Here's how the part is built. I have some questions about the finished solid (model axes, mm). Face numbers are marked on the shaded views. A direction names the side the tool comes from. Give positions to 0.01 mm unless a question says otherwise; leave off trailing zeros. Loops run counter-clockwise (first coordinate to the right, second up) from the corner with the lowest first, then second, coordinate; pieces in that order, holes last. Notation, with made-up numbers: M 52,85 L 110,85 A21 ccw 110,122 Z; hole C 26.5,-11 d10. An arc over 180 degrees is marked long. Write item = value, one per line. Start each with the question number.
```python
from build123d import *

# Parameters (mm, degrees)
SKETCH1_R      = 5
EXTRUDE1_DEPTH = 68
SKETCH2_R      = 2.25
EXTRUDE2_DEPTH = 68


with BuildPart() as part:
    # Sketch1 → Extrude1 (new body)
    with BuildSketch(Plane.XY):
        Polygon((-18.5, -8), (-10, -8), (-5, -13), (5, -13), (10, -8), (18.5, -8), (18.5, 3.5), (20, 5), (20, 13), (9, 13), (8, 12), (-8, 12), (-9, 13), (-20, 13), (-20, 5), (-18.5, 3.5), align=None)
        Circle(SKETCH1_R, mode=Mode.SUBTRACT)
    extrude(amount=EXTRUDE1_DEPTH)

    # Sketch2 → Extrude2 (cut)
    with BuildSketch(Plane(origin=(0, 13, 0), x_dir=(1, 0, 0), z_dir=(0, 1, 0))):
        with Locations((-14, -11.2)):
            Circle(SKETCH2_R)
        with Locations((14, -11.2)):
            Circle(SKETCH2_R)
        with Locations((14, -56.8)):
            Circle(SKETCH2_R)
        with Locations((-14, -56.8)):
            Circle(SKETCH2_R)
    extrude(amount=-EXTRUDE2_DEPTH, mode=Mode.SUBTRACT)


solid = part.part
```
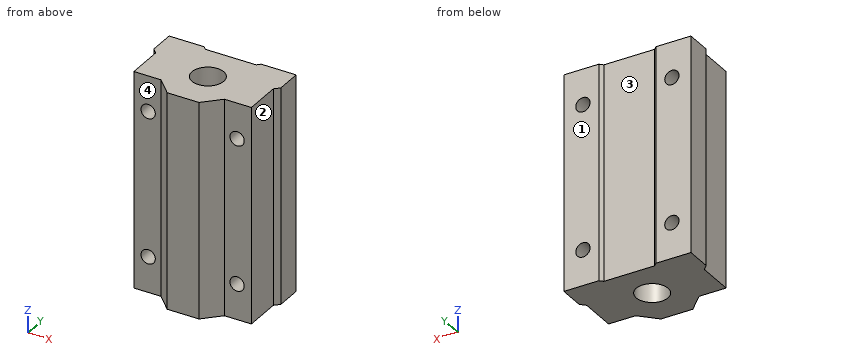
Q1. Will these pins go through, and if not, where does the flat tip stop? pin 1 (4 mm diameter, centred on x = -14, z = 11.2, fed in from +Y) (3 decimals); pin 2 (3.5 mm diameter, centred on y = -2.5, z = 17.5, fed in from +X); pin 3 (4 mm diameter, centred on x = 13.5, z = 30.5, fed in from -Y); pin 4 (9 mm diameter, centred on y = -3.5, z = 47, fed in from -X).
Q2. If I drill on line 1 along Z through (x, y) = (-14, -2.5); line 2 along X through (y, z) = (5.75, 10); line 3 along Z through (x, y) = (15.5, -4.75), over which ranges is the centre line in solid material (lowest first)?
Q3. If we section it at D-D, the plane x = -14: List the corners of the cut face in (y, z) for me.
Q4. If we section it at A-A, the plane z = 11.2: List the corners of the cut face in (x, y) for me, then the cut area to 3 significant figures.
Q5. On a 3-axis mill with a long thin cutter (end or side, diameter ignored), from which of +Z, -Z, +X, -X, +Y, -Y can I reach the whole of each face in a straight line? I mean the marked faces 1, 2, 3 and 4. Say none if no direction works.
Q6. If we section it at B-B, the plane y = 7: List the corners of the cut face in (x, z) for me.
Q7. If we section it at C-C, the plane z = 24.5: List the corners of the cut face in (x, y) for me, then the cut area to 3 significant figures.
Resolved:
q1.pin_1 = through
q1.pin_2 = 18.5
q1.pin_3 = -8
q1.pin_4 = -18.5
q2.line_1 = 0 to 8.95, 13.45 to 54.55, 59.05 to 68
q2.line_2 = -20 to -15.9, -12.1 to 12.1, 15.9 to 20
q2.line_3 = 0 to 9.52, 12.88 to 55.12, 58.48 to 68
q3.outline = M -8,0 L 13,0 L 13,8.95 L -8,8.95 Z; M -8,13.45 L 13,13.45 L 13,54.55 L -8,54.55 Z; M -8,59.05 L 13,59.05 L 13,68 L -8,68 Z
q4.outline = M -20,5 L -18.5,3.5 L -18.5,-8 L -16.25,-8 L -16.25,13 L -20,13 Z; M -11.75,-8 L -10,-8 L -5,-13 L 5,-13 L 10,-8 L 11.75,-8 L 11.75,13 L 9,13 L 8,12 L -8,12 L -9,13 L -11.75,13 Z; M 16.25,-8 L 18.5,-8 L 18.5,3.5 L 20,5 L 20,13 L 16.25,13 Z; hole C 0,0 d10
q4.area = 594 mm²
q5.face_1 = +Z, -Z, +X, -X, +Y
q5.face_2 = +Z, -Z, +X, -Y
q5.face_3 = +Z, -Z, +Y
q5.face_4 = +Z, -Z, -X, -Y
q6.outline = M -20,0 L 20,0 L 20,68 L -20,68 Z; hole C -14,11.2 d4.5; hole C -14,56.8 d4.5; hole C 14,11.2 d4.5; hole C 14,56.8 d4.5
q7.outline = M -20,5 L -18.5,3.5 L -18.5,-8 L -10,-8 L -5,-13 L 5,-13 L 10,-8 L 18.5,-8 L 18.5,3.5 L 20,5 L 20,13 L 9,13 L 8,12 L -8,12 L -9,13 L -20,13 Z; hole C 0,0 d10
q7.area = 783 mm²
